Verification items for the finished model (mm, model axes). Face numbers are marked on the shaded views. A direction names the side the tool comes from. Round coordinates to 2 decimals unless told otherwise and drop trailing zeros. Order: outer loops, then holes, each group sorted by start corner. A loop starts at its lowest first (then second) coordinate and runs counter-clockwise, first axis right, second up. Notation, with made-up numbers: (86, 4.5) -> (113, 4.5) arc R18 cw to (113, 18.5) -> close; hole circle Ø3 at (49.5, -26). An arc over 180 degrees is marked (long way). Put each result on its own line as item: value.
from build123d import *

# Parameters (mm, degrees)
BOSS_EXTRUDE1_DEPTH = 26
BOSS_EXTRUDE2_DEPTH = 2
BOSS_EXTRUDE3_DEPTH = 2
CUT_EXTRUDE1_DEPTH  = 4
CUT_EXTRUDE2_DEPTH  = 4


with BuildPart() as part:
    # Sketch1 → Boss-Extrude1 (new body)
    with BuildSketch(Plane(origin=(0, 0, 0), x_dir=(1, 0, 0), z_dir=(0, 1, 0))):
        Polygon((0, 0), (0, 35), (3, 35), (3, 3), (35, 3), (35, 0), align=None)
    extrude(amount=BOSS_EXTRUDE1_DEPTH)

    # Sketch2 → Boss-Extrude2 (add)
    with BuildSketch(Plane(origin=(0, 26, 0), x_dir=(1, 0, 0), z_dir=(0, 1, 0))):
        Polygon((3, 35), (0, 35), (0, 0), (35, 0), (35, 3), (31, 3), (3, 31), align=None)
    extrude(amount=BOSS_EXTRUDE2_DEPTH)

    # Sketch3 → Boss-Extrude3 (add)
    with BuildSketch(Plane.XZ):
        Polygon((0, 0), (0, -35), (3, -35), (3, -31), (31, -3), (35, -3), (35, 0), align=None)
    extrude(amount=BOSS_EXTRUDE3_DEPTH)

    # Sketch4 → Cut-Extrude1 (cut, through all)
    with BuildSketch(Plane(origin=(0, 0, -3), x_dir=(-1, 0, 0), z_dir=(0, 0, -1))):
        with BuildLine():
            Line((-27, 16.4), (-8, 16.4))
            ThreePointArc((-8, 16.4), (-4.6, 13), (-8, 9.6))
            Line((-8, 9.6), (-27, 9.6))
            ThreePointArc((-27, 9.6), (-30.4, 13), (-27, 16.4))
        make_face()
    extrude(amount=-CUT_EXTRUDE1_DEPTH, mode=Mode.SUBTRACT)

    # Sketch5 → Cut-Extrude2 (cut, through all)
    with BuildSketch(Plane(origin=(3, 0, 0), x_dir=(0, 0, -1), z_dir=(1, 0, 0))):
        with BuildLine():
            Line((8, 16.4), (27, 16.4))
            ThreePointArc((27, 16.4), (30.4, 13), (27, 9.6))
            Line((27, 9.6), (8, 9.6))
            ThreePointArc((8, 9.6), (4.6, 13), (8, 16.4))
        make_face()
    extrude(amount=-CUT_EXTRUDE2_DEPTH, mode=Mode.SUBTRACT)


solid = part.part
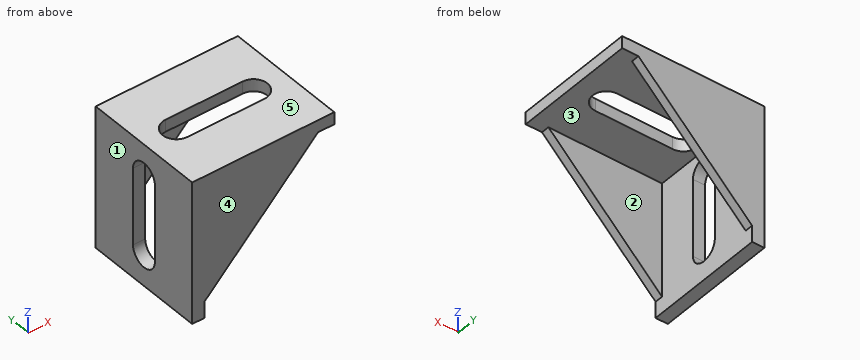
Item 1: Release check for a two-part mould opening along Z. For the marked faces 3, 4 and 5 record: +Z half, -Z half, draft (parallel to the pull), parting line (faces both ways), or undercut.
Check sheet entries:
face 3: -Z half
face 4: draft
face 5: +Z half
Item 2: Section check B-B on z = -24. Record the boundary of the cut face in (x, y), then the cut area to 3 significant figures.
Check sheet entries:
outline: (0, -2) -> (10, -2) -> (10, 0) -> (3, 0) -> (3, 9.6) -> (0, 9.6) -> close; (0, 16.4) -> (3, 16.4) -> (3, 26) -> (10, 26) -> (10, 28) -> (0, 28) -> close
area: 97.6 mm^2
Item 3: Section check C-C on y = 0.75. Record the boundary of the cut face in (x, z).
Check sheet entries:
outline: (0, -35) -> (3, -35) -> (3, -3) -> (35, -3) -> (35, 0) -> (0, 0) -> close
Item 4: Material ranges on L1, parallel to Y at x = 23.5, z = -5; L2, parallel to Y at x = 23, z = -2.5; L3, parallel to Z at x = 26, y = 18.5, recorded low to high. Write a range as [from, to].
Check sheet entries:
L1: y = [-2, 0], [26, 28]
L2: y = [-2, 9.6], [16.4, 28]
L3: z = [-3, 0]
Item 5: Section check A-A on y = 13. Record the boundary of the cut face in (x, z).
Check sheet entries:
outline: (0, -35) -> (3, -35) -> (3, -30.4) -> (0, -30.4) -> close; (0, -4.6) -> (3, -4.6) -> (3, -3) -> (4.6, -3) -> (4.6, 0) -> (0, 0) -> close; (30.4, -3) -> (35, -3) -> (35, 0) -> (30.4, 0) -> close
Item 6: Section check D-D on z = -9. Record the boundary of the cut face in (x, y).
Check sheet entries:
outline: (0, -2) -> (25, -2) -> (25, 0) -> (3, 0) -> (3, 9.6) -> (0, 9.6) -> close; (0, 16.4) -> (3, 16.4) -> (3, 26) -> (25, 26) -> (25, 28) -> (0, 28) -> close
Item 7: Tool access check on the marked faces 1 and 2. Record the directions out of +Z, -Z, +X, -X, +Y, -Y that give a thin tool (end or side, any length) a straight path to the whole face; none if there is none.
Check sheet entries:
face 1: +Z, -Z, -X, +Y, -Y
face 2: -Z, +X
Item 8: Gauge pin test, flat end, axial feed: pin 1 Ø1.5 at (y, z) = (22.5, -18.5) entering from +X. Record the tip position at first contact, or that the pin passes through.
Check sheet entries:
pin 1: stops at x = 3
